Autodesk Inventor part; units mm, degrees
ref_plane "YZ Plane" through (0, 0, 0) normal (1, 0, 0) x (0, 1, 0)
ref_plane "XZ Plane" through (0, 0, 0) normal (0, 1, 0) x (-1, 0, 0)
ref_plane "XY Plane" through (0, 0, 0) normal (0, 0, 1) x (1, 0, 0)
sketch "Sketch1" plane through (0, 0, 0) normal (0, 1, 0) x (-1, 0, 0)
  line L0 (0, 0) -> (20, 0)
  line L1 (20, 0) -> (20, -40)
  line L2 (20, -40) -> (0, -40)
  line L3 (0, -40) -> (0, 0)
  dimension "d0" = 40
  dimension "d1" = 20
extrude "Extrusion1" add sketch "Sketch1" along normal blind 24.7
sketch "Sketch2" plane through (0, 24.7, 0) normal (0, 1, 0) x (1, 0, 0)
  line L0 (0, -8) -> (-20, -8)
  line L1 (-20, -8) -> (-20, 48)
  line L2 (-20, 48) -> (0, 48)
  line L3 (0, 48) -> (0, -8)
  line L4 (-20, 40) -> (-20, 0)
  line L5 (-20, 0) -> (0, 0)
  dimension "d4" = 56
  dimension "d5" = 20
  dimension "d6" = 0
  dimension "d7" = 8
extrude "Extrusion2" add sketch "Sketch2" along normal blind 2.7
sketch "Sketch3" plane through (0, 27.4, 0) normal (0, 1, 0) x (1, 0, 0)
  line L0 (-20, 48) -> (-20, 40)
  line L1 (0, 0) -> (-20, 0)
  line L2 (-20, 0) -> (-20, 40)
  line L3 (-20, 40) -> (0, 40)
  line L4 (0, 40) -> (0, 0)
extrude "Extrusion3" add sketch "Sketch3" along normal blind 10.1
sketch "Sketch4" plane through (0, 37.5, 0) normal (0, 1, 0) x (1, 0, 0)
  circle A0 centre (-10, 27.5) radius 2.5
  line L0 (0, 40) -> (-20, 40)
  line L1 (0, 0) -> (0, 40)
  dimension "d12" = 12.5
  dimension "d13" = 5
  dimension "d16" = 10
extrude "Extrusion4" add sketch "Sketch4" along normal blind 4
sketch "Sketch5" plane through (0, 27.4, 0) normal (0, 1, 0) x (1, 0, 0)
  circle A0 centre (-5, -4) radius 2.5
  circle A1 centre (-15, -4) radius 2.5
  line L0 (-20, 0) -> (-20, -8)
  line L1 (0, -8) -> (0, 0)
  line L2 (-20, -8) -> (0, -8)
  line L3 (17.0621, 20) -> (-50.3662, 20) construction
  line L4 (-20, 0) -> (0, 0)
  circle A2 centre (-5, 44) radius 2.5
  circle A3 centre (-15, 44) radius 2.5
  dimension "d17" = 5
  dimension "d18" = 5
  dimension "d19" = 5
  dimension "d20" = 4
  dimension "d21" = 4
  dimension "d22" = 20
extrude "Extrusion5" cut sketch "Sketch5" against normal blind 4 contours A0 | A1 | A2 | A3
equation "\"d21\" = d20"
properties part number "motor"
Work out the finished part from the listing and answer in its coordinate system (mm). A direction names the side the tool comes from. Coordinates: 2 decimals unless noted, no trailing zeros. Write each loop counter-clockwise with the first axis right and the second up, starting at its lowest first coordinate (ties: lowest second). Pieces come first, ordered by that corner, then holes. Notation, with made-up numbers: (13, -22) - (45, -22) arc R22 ccw to (45, -5) - close; hole circle Ø1 at (82.5, 5.5). An arc over 180 degrees is marked (long way). Answer as a JSON object with one key per item and string values.
Q1. Find section D-D (y = 12). Write down the section's boundary in (x, z), plus the area to 3 significant figures.
Results list:
{"outline": "(-20, -40) - (0, -40) - (0, 0) - (-20, 0) - close", "area": "800 mm^2"}
Q2. Given pin 1 Ø10 at (x, y) = (-12, 10) entering from +Z; pin 2 Ø5 at (x, y) = (-5.5, 34) entering from -Z; pin 3 Ø2.5 at (x, z) = (-15, -42) entering from +Y; pin 4 Ø4 at (x, z) = (-5, 4) entering from +Y, each flat-ended and moving along its own axis, determine where each tip first touches the part or whether it passes through.
Results list:
{"pin 1": "stops at z = 0", "pin 2": "stops at z = -40", "pin 3": "stops at y = 27.4", "pin 4": "passes through"}
Q3. Find section C-C (x = -18.5). Write down the section's boundary in (y, z).
Results list:
{"outline": "(0, -40) - (24.7, -40) - (24.7, -48) - (27.4, -48) - (27.4, -40) - (37.5, -40) - (37.5, 0) - (27.4, 0) - (27.4, 8) - (24.7, 8) - (24.7, 0) - (0, 0) - close"}
Q4. Which of the six approach directions +Z, -Z, +X, -X, +Y, -Y give full straight-line access (tool end or side, diameter ignored) to faces 5 (the flat face through (-10, 27.4, 4)), 6 (the cylindrical face through (-10, 39, -25)), 7 (the flat face through (-10, 12, -40)), 8 (the flat face through (-10, 24.7, 4))?
Results list:
{"face 5": "+Z, +X, -X, +Y", "face 6": "+Y", "face 7": "-Z, +X, -X, -Y", "face 8": "+Z, +X, -X, -Y"}
Q5. Find section B-B (x = -13.5). Write down the section's boundary in (y, z).
Results list:
{"outline": "(0, -40) - (24.7, -40) - (24.7, -42) - (27.4, -42) - (27.4, -40) - (37.5, -40) - (37.5, 0) - (27.4, 0) - (27.4, 2) - (24.7, 2) - (24.7, 0) - (0, 0) - close; (24.7, -48) - (27.4, -48) - (27.4, -46) - (24.7, -46) - close; (24.7, 6) - (27.4, 6) - (27.4, 8) - (24.7, 8) - close"}
Q6. For a pull along X with two mould halves and no side action, classify faces 1 (the flat face through (0, 18, -20)), 2 (the flat face through (-10, 37.5, -20)), 3 (the cylindrical face through (-15.54, 26.07, -41.56)), 4 (the cylindrical face through (-16.84, 26.07, 2.31)) as pulls with the +X half, pulls with the -X half, needs draft (parallel to the pull), parting line crosses it, or undercut.
Results list:
{"face 1": "pulls with the +X half", "face 2": "needs draft", "face 3": "undercut", "face 4": "undercut"}
Q7. Consider L1, parallel to X at y = 25.35, z = 4; L2, parallel to Z at x = -5, y = 26.3; L3, parallel to Z at x = -3.5, y = 2. Determine where each line is inside the solid, lowest interval first. Write a range as from..to.
Results list:
{"L1": "x = -20..-17.5, -12.5..-7.5, -2.5..0", "L2": "z = -48..-46.5, -41.5..1.5, 6.5..8", "L3": "z = -40..0"}
Q8. Find section A-A (z = -44). Write down the section's boundary in (x, y), plus the area to 3 significant figures.
Results list:
{"outline": "(-20, 24.7) - (-17.5, 24.7) - (-17.5, 27.4) - (-20, 27.4) - close; (-12.5, 24.7) - (-7.5, 24.7) - (-7.5, 27.4) - (-12.5, 27.4) - close; (-2.5, 24.7) - (0, 24.7) - (0, 27.4) - (-2.5, 27.4) - close", "area": "27.0 mm^2"}
